```python
from build123d import *

# Parameters (mm, degrees)
SKETCH1_R           = 1.5
BOSS_EXTRUDE1_DEPTH = 6
BOSS_EXTRUDE2_DEPTH = 10
SKETCH3_R           = 1.5
CUT_EXTRUDE1_DEPTH  = 6


with BuildPart() as part:
    # Sketch1 → Boss-Extrude1 (new body)
    with BuildSketch(Plane.XY):
        Circle(SKETCH1_R)
    extrude(amount=BOSS_EXTRUDE1_DEPTH)

    # Sketch2 → Boss-Extrude2 (add)
    with BuildSketch(Plane(origin=(0, 0, 0), x_dir=(-1, 0, 0), z_dir=(0, 0, -1))):
        Polygon((1.299038106, 2.25), (-1.299038106, 2.25), (-2.598076211, 0), (-1.299038106, -2.25), (1.299038106, -2.25), (2.598076211, 0), align=None)
    extrude(amount=BOSS_EXTRUDE2_DEPTH)

    # Sketch3 → Cut-Extrude1 (cut)
    with BuildSketch(Plane(origin=(0, 0, -10), x_dir=(-1, 0, 0), z_dir=(0, 0, -1))):
        Circle(SKETCH3_R)
    extrude(amount=-CUT_EXTRUDE1_DEPTH, mode=Mode.SUBTRACT)


solid = part.part
```
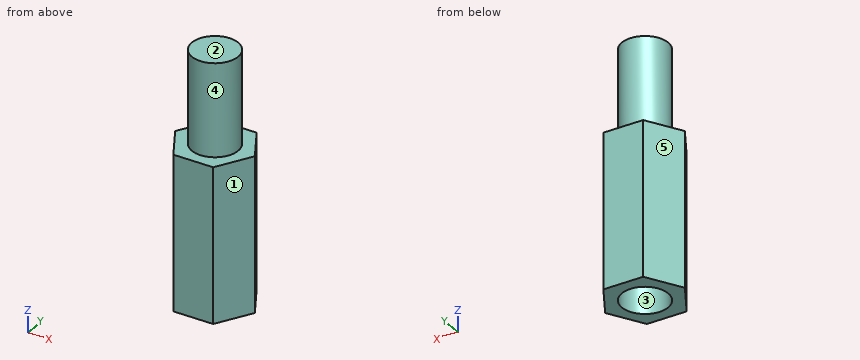
Can you work these out from the model? Positions are in its coordinate system, mm. Face numbers are marked on the shaded views. A direction names the side the tool comes from. Coordinates: 2 decimals unless noted, no trailing zeros. Write each loop counter-clockwise with the first axis right and the second up, starting at its lowest first coordinate (ties: lowest second). Pieces come first, ordered by that corner, then holes. Notation, with made-up numbers: (-20, 14) - (15, 14) arc R7 cw to (15, 24) - close; hole circle Ø6 at (-6.75, 19.5). An arc over 180 degrees is marked (long way). Return JSON: item names as keys, results as strings.
Q1. If we section it at D-D (y = 0.45): Please give me the cut outline in (x, z), then the cut area to 3 significant figures.
Computed values:
{"outline": "(-2.34, -10) - (-1.43, -10) - (-1.43, -4) - (1.43, -4) - (1.43, -10) - (2.34, -10) - (2.34, 0) - (1.43, 0) - (1.43, 6) - (-1.43, 6) - (-1.43, 0) - (-2.34, 0) - close", "area": "46.8 mm2"}
Q2. Thinking about a two-plate mould opening in Y: for the marked faces 1, 2 and 3, which applies, +Y half, -Y half, draft (parallel to the pull), parting line (faces both ways), or undercut?
Computed values:
{"face 1": "-Y half", "face 2": "draft", "face 3": "undercut"}
Q3. Please list where these lines run through material, in increasing order: L1, parallel to Y at x = 0, z = -5.5; L2, parallel to Z at x = -0.2, y = 1.75; L3, parallel to Z at x = 0.95, y = 0.8. Write a range as from..to.
Computed values:
{"L1": "y = -2.25..-1.5, 1.5..2.25", "L2": "z = -10..0", "L3": "z = -4..6"}
Q4. I'm going to push flat-ended pins straight in: pin 1 Ø1 at (y, z) = (1, -6) entering from +X; pin 2 Ø1.5 at (x, y) = (0, 0.5) entering from -Z. Where does each tip first touch, or does it pass through?
Computed values:
{"pin 1": "stops at x = 2.31", "pin 2": "stops at z = -4"}
Q5. If we section it at B-B (z = -2.5): Please give me the cut outline in (x, y), then the cut area to 3 significant figures.
Computed values:
{"outline": "(-2.6, 0) - (-1.3, -2.25) - (1.3, -2.25) - (2.6, 0) - (1.3, 2.25) - (-1.3, 2.25) - close", "area": "17.5 mm2"}
Q6. If we section it at C-C (x = 1.05): Please give me the cut outline in (y, z), then the cut area to 3 significant figures.
Computed values:
{"outline": "(-2.25, -10) - (-1.07, -10) - (-1.07, -4) - (1.07, -4) - (1.07, -10) - (2.25, -10) - (2.25, 0) - (1.07, 0) - (1.07, 6) - (-1.07, 6) - (-1.07, 0) - (-2.25, 0) - close", "area": "45.0 mm2"}
Q7. If we section it at A-A (z = -7): Please give me the cut outline in (x, y), then the cut area to 3 significant figures.
Computed values:
{"outline": "(-2.6, 0) - (-1.3, -2.25) - (1.3, -2.25) - (2.6, 0) - (1.3, 2.25) - (-1.3, 2.25) - close; hole circle Ø3 at (0, 0)", "area": "10.5 mm2"}
Q8. On a 3-axis mill with a long thin cutter (end or side, diameter ignored), from which of +Z, -Z, +X, -X, +Y, -Y can I reach the whole of each face in a straight line? I mean the marked faces 4 and 5. Say none if no direction works.
Computed values:
{"face 4": "+Z", "face 5": "+Z, -Z, -X, +Y"}
